Verification items for the finished model (mm, model axes). Coordinates: 2 decimals unless noted, no trailing zeros. Order: outer loops, then holes, each group sorted by start corner. A loop starts at its lowest first (then second) coordinate and runs counter-clockwise, first axis right, second up. Notation, with made-up numbers: M 19,-19.75 L 39,-19.75 A21 ccw 39,-14.75 Z; hole C -12,40.25 d7. An arc over 180 degrees is marked long. Answer as a JSON object with one key per item and string values. Group by question number.
(1) Gauge pin test, flat ends, axial feed: pin 1 Ø3.5 at (x, z) = (140, -65) entering from -Y; pin 2 Ø1 at (x, y) = (57, 1) entering from +Z. Record the tip position at first contact, or that the pin passes through.
(2) Cross-section at C-C (y = 0.3). Count the separate pieces of the cut face and the enclosed holes in it, plus the area to 3 significant figures.
(3) Mould release check, pull along X, two halves, no side actions. Record for faces 1 (the face through (6.45, 0.83, 4.94)), 2 (the face through (72, 0, -22)): released by +X, released by -X, zero draft, split by the parting line, or undercut.
(4) Material ranges on line 1 (Z direction, x = 5, y = 0.8); line 2 (Z direction, x = 128.5, y = 0.25); line 3 (X direction, y = 1, z = -65), recorded low to high.
(5) Cross-section at D-D (z = -65). Enter the section's corners in (x, y) (3 decimals), plus the area to 3 significant figures.
(6) Cross-section at B-B (x = 58). Enter the section's corners in (y, z).
(7) Cross-section at A-A (z = -49). Enter the section's corners in (x, y), plus the area to 3 significant figures.
from build123d import *

# Parameters (mm, degrees)
EXTRUDE_1_DEPTH                = 2
HOLE_WIZARD_M3_5_2_D           = 2.9
HOLE_WIZARD_M3_5_2_CSINK_D     = 3.55
HOLE_WIZARD_M3_5_2_CSINK_ANGLE = 90
CUT_EXTRUDE_1_DEPTH            = 3
SKETCH_7_W                     = 125
SKETCH_7_H                     = 45.551843708
CUT_EXTRUDE_2_DEPTH            = 3


with BuildPart() as part:
    # 草图1 → 凸台-拉伸1 (new body)
    with BuildSketch(Plane(origin=(0, 0, 0), x_dir=(1, 0, 0), z_dir=(0, 1, 0))):
        Polygon((0, 0), (0, -10), (15, -10), (15, 0), (15, 10), (130, 10), (130, 0), (130, -10), (145, -10), (145, 0), (145, 80), (0, 80), align=None)
    extrude(amount=EXTRUDE_1_DEPTH)

    # M3.5 螺纹孔2 (through all)
    with Locations(Plane(origin=(0, 2, 0), x_dir=(1, 0, 0), z_dir=(0, 1, 0))):
        with Locations((5, 65), (5, 75), (140, 75), (140, -5), (5, -5), (140, 65)):
            CounterSinkHole(HOLE_WIZARD_M3_5_2_D / 2, HOLE_WIZARD_M3_5_2_CSINK_D / 2, counter_sink_angle=HOLE_WIZARD_M3_5_2_CSINK_ANGLE)

    # 草图6 → 切除-拉伸1 (cut)
    with BuildSketch(Plane(origin=(0, 2, 0), x_dir=(1, 0, 0), z_dir=(0, 1, 0))):
        with BuildLine():
            Line((12, 19), (133, 19))
            ThreePointArc((133, 19), (135, 17), (133, 15))
            Line((133, 15), (12, 15))
            ThreePointArc((12, 15), (10, 17), (12, 19))
        make_face()
    extrude(amount=-CUT_EXTRUDE_1_DEPTH, mode=Mode.SUBTRACT)

    # 草图7 → 切除-拉伸2 (cut)
    with BuildSketch(Plane(origin=(0, 2, 0), x_dir=(1, 0, 0), z_dir=(0, 1, 0))):
        with Locations((72.5, 45.7539171)):
            Rectangle(SKETCH_7_W, SKETCH_7_H)
    extrude(amount=-CUT_EXTRUDE_2_DEPTH, mode=Mode.SUBTRACT)


solid = part.part
Taken from the geometry:
{
 "1": {"pin 1": "stops at y = 0", "pin 2": "stops at z = -10"},
 "2": {"separate pieces": "1", "enclosed holes": "8", "area": "4,520 mm²"},
 "3": {"face 1": "undercut", "face 2": "zero draft"},
 "4": {"line 1": "z = -80 to -76.45, -73.55 to -66.45, -63.55 to 3.55, 6.45 to 10", "line 2": "z = -80 to -68.53, -22.98 to -19, -15 to -10", "line 3": "x = 0 to 3.55, 6.45 to 10, 135 to 138.55, 141.45 to 145"},
 "5": {"outline": "M 0,0 L 3.55,0 L 3.55,1.675 L 3.225,2 L 0,2 Z; M 6.45,0 L 10,0 L 10,2 L 6.775,2 L 6.45,1.675 Z; M 135,0 L 138.55,0 L 138.55,1.675 L 138.225,2 L 135,2 Z; M 141.45,0 L 145,0 L 145,2 L 141.775,2 L 141.45,1.675 Z", "area": "28.2 mm²"},
 "6": {"outline": "M 0,-80 L 2,-80 L 2,-68.53 L 0,-68.53 Z; M 0,-22.98 L 2,-22.98 L 2,-19 L 0,-19 Z; M 0,-15 L 2,-15 L 2,-10 L 0,-10 Z"},
 "7": {"outline": "M 0,0 L 10,0 L 10,2 L 0,2 Z; M 135,0 L 145,0 L 145,2 L 135,2 Z", "area": "40.0 mm²"}
}
